```python
from build123d import *

# Parameters (mm, degrees)
F0_R      = 75
F1_DEPTH  = 30
F2_R      = 5
F3_R      = 5
F4_R      = 62.5
F5_DEPTH  = 30
F7_E2_W   = 124.9627603046
F7_E2_H   = 30
F8_DEPTH  = 4
F10_E3_W  = 124.8690485954
F10_E3_H  = 30
F11_DEPTH = 4
F12_R     = 1
F13_DEPTH = 12
F14_R     = 1
F15_DEPTH = 12


with BuildPart() as f1:
    # F0 (on Top) → F1 (new body)
    with BuildSketch(Plane.XY):
        with Locations((-35.8805991709, 25.7855858654)):
            Circle(F0_R)
    extrude(amount=F1_DEPTH)

    # F2
    f2_edges = [f1.edges().sort_by_distance(p)[0] for p in [
        (-110.880599, 25.785586, 0),
    ]]
    fillet(f2_edges, radius=F2_R)

    # F3
    f3_edges = [f1.edges().sort_by_distance(p)[0] for p in [
        (-110.880599, 25.785586, 30),
    ]]
    fillet(f3_edges, radius=F3_R)

    # F4 (on face) → F5 (cut)
    with BuildSketch(Plane(origin=(0, 0, 0), x_dir=(1, 0, 0), z_dir=(0, 0, -1))):
        with Locations((-35.8805991709, -25.7855858654)):
            Circle(F4_R)
    extrude(amount=-F5_DEPTH, mode=Mode.SUBTRACT)

    # F7_E2 (on explicit) → F8 (join, symmetric)
    with BuildSketch(Plane(origin=(-34.3551044097, 88.2669660177, 0), x_dir=(0, -1, 0), z_dir=(-1, 0, 0))):
        with Locations((62.4813801523, 15)):
            Rectangle(F7_E2_W, F7_E2_H)
    extrude(amount=F8_DEPTH, both=True)

    # F10_E3 (on explicit) → F11 (join, symmetric)
    with BuildSketch(Plane(origin=(-98.322533071, 25.6824456155, 0), x_dir=(1, 0, 0), z_dir=(0, -1, 0))):
        with Locations((62.4345242977, 15)):
            Rectangle(F10_E3_W, F10_E3_H)
    extrude(amount=F11_DEPTH, both=True)

    # F12 (on face) → F13 (cut)
    with BuildSketch(Plane.XY.offset(30)):
        with Locations((-34.3549661338, 25.6826244295)):
            Circle(F12_R)
    extrude(amount=-F13_DEPTH, mode=Mode.SUBTRACT)

    # F14 (on Top) → F15 (cut)
    with BuildSketch(Plane.XY):
        with Locations((-34.3551188707, 25.6825555116)):
            Circle(F14_R)
    extrude(amount=F15_DEPTH, mode=Mode.SUBTRACT)


solid = f1.part
```
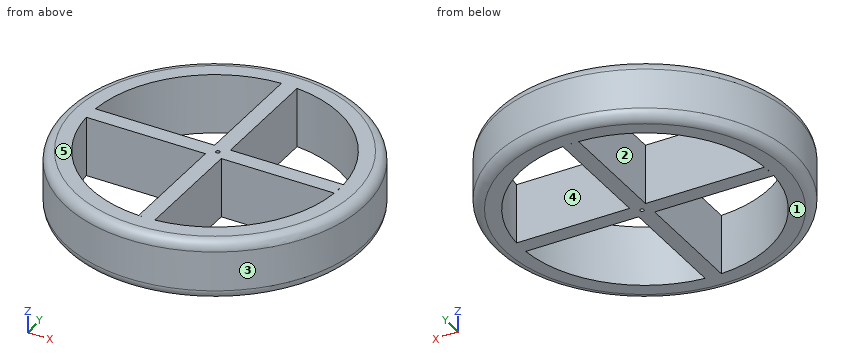
Design review of the part built by this model. Coordinates are the model's own, in mm. Face numbers are marked on the shaded views. A direction names the side the tool comes from. Coordinates: 2 decimals unless noted, no trailing zeros. Answer as a JSON object with one key per item and string values.
Q1. Take a section at A-A on z = 7.5. Give the number of separate pieces and of enclosed holes in the cut face, plus the area to 3 significant figures.
Answer block:
{"separate pieces": "1", "enclosed holes": "9", "area": "7,330 mm^2"}
Q2. Clearance check with flat-ended pins moving along their axes: pin 1 Ø3 at (y, z) = (63.5, 8) entering from -X; pin 2 Ø1.6 at (x, y) = (-34, 25.5) entering from +Z; pin 3 Ø10 at (y, z) = (-26, 25.5) entering from -X; pin 4 Ø15 at (x, z) = (3, 12) entering from +Y (3 decimals). State where each tip first meets the part, or that it passes through.
Answer block:
{"pin 1": "stops at x = -101.56", "pin 2": "stops at z = 30", "pin 3": "stops at x = -94.49", "pin 4": "stops at y = 93.905"}
Q3. To check wall thickness, follow L1, parallel to X at y = 45.5, z = 13.75; L2, parallel to X at y = 61.5, z = 17; L3, parallel to Y at x = -18.5, z = 9.5. State the ranges of each line that lie inside material, in increasing order.
Answer block:
{"L1": "x = -108.24 to -95.19, -38.36 to -30.36, 23.43 to 36.48", "L2": "x = -101.83 to -87.17, -38.36 to -30.36, 15.41 to 30.07", "L3": "y = -47.17 to -34.25, 21.68 to 29.68, 85.82 to 98.74"}
Q4. Tool access review of the marked faces 4 and 5: name each direction out of +Z, -Z, +X, -X, +Y, -Y from which nothing blocks a thin tool from reaching the whole face with its end or side.
Answer block:
{"face 4": "+Z, -Z", "face 5": "+Z, +X, -X, +Y, -Y"}
Q5. The part is to be moulded in two halves that separate along X. For the marked faces 1, 2 and 3, say which applies: +X half, -X half, draft (parallel to the pull), parting line (faces both ways), or undercut.
Answer block:
{"face 1": "draft", "face 2": "undercut", "face 3": "parting line"}
